Can you work these out from the model? Positions are in its coordinate system, mm. A direction names the side the tool comes from. Give positions to 0.01 mm unless a question says otherwise; leave off trailing zeros. Order: outer loops, then holes, each group sorted by start corner. A loop starts at its lowest first (then second) coordinate and runs counter-clockwise, first axis right, second up.
Item 1: If I drill on line 1 along X through (y, z) = (2.85, -114.5); line 2 along Z through (x, y) = (2.25, -0.5); line 3 along X through (y, z) = (3, -115.5), over which ranges is the centre line in solid material (lowest first)?
Item 2: I'm going to push flat-ended pins straight in: pin 1 Ø1.8 at (x, z) = (6, -114.5) entering from -Y; pin 2 Ø4 at (x, z) = (3, -114) entering from -Y; pin 3 Ø1.6 at (x, y) = (4, 1) entering from -Z; pin 4 Ø0.8 at (x, z) = (5, -109.5) entering from -Y. Where does each tip first touch, or does it pass through?
Item 3: I want a section at D-D, the plane z = -114.5. Write out the boundary of the cut face in (x, y).
Item 4: I want a section at A-A, the plane x = 0. Write out the boundary of the cut face in (y, z), then the cut area to 3 significant figures.
Item 5: If we mould it in two halves opening along X, with no side actions, what happens to faces 1 (the flat face through (3, 4, -113)), 2 (the flat face through (-3, 1.2, -109.5)), 3 (the cylindrical face through (0, 3, -115.6)), 4 (the flat face through (9, 1.2, -109.5))? For each: +X half, -X half, draft (parallel to the pull), parting line (faces both ways), or undercut.
Item 6: I want a section at B-B, the plane y = -0.5. Write out the boundary of the cut face in (x, z).
Item 7: I want a section at C-C, the plane x = 3.5. Write out the boundary of the cut face in (y, z), then the cut area to 3 significant figures.
Item 8: Which directions (+Z, -Z, +X, -X, +Y, -Y) give clear straight access to the entire face, cutting with the end or side of a thin tool? Please do faces 5 (the flat face through (3, 3, -106.5)), 6 (the flat face through (3, 2, -114)), 7 (the cylindrical face through (2.916, 0.432, -106.985)).
```python
from build123d import *

# Parameters (mm, degrees)
SKETCH_1_W                      = 9.5
SKETCH_1_H                      = 13.25
EXTRUDE_1_DEPTH                 = 2
EXTRUDE_2_DEPTH                 = 12
PATTERN_LINEAR_1_COUNT          = 5
PATTERN_LINEAR_1_PITCH          = 22
HOLE_WIZARD_2_2_2_2_1_D         = 2.1
EXTRUDE_3_DEPTH                 = 12
SKETCH_7_W                      = 1.05
SKETCH_7_H                      = 15
EXTRUDE_4_DEPTH                 = 110
HOLE_WIZARD_2_0_2_2_D           = 2
HOLE_WIZARD_2_0_2_2_ON_FACE_2_D = 2
CUT_EXTRUDE_1_DEPTH             = 135.480746763
CUT_EXTRUDE_1_DEPTH_BACK        = 135.480746763
SKETCH_14_W                     = 52.846717088
SKETCH_14_H                     = 8
SKETCH19_W                      = 12
SKETCH19_H                      = 12
EXTRUDE23_DEPTH                 = 2
SKETCH20_R                      = 1.1
EXTRUDE24_DEPTH                 = 2
CUT_EXTRUDE_2_DEPTH             = 22
CUT_EXTRUDE_2_DEPTH_BACK        = 24
SKETCH_15_W                     = 124.248356878
SKETCH_15_H                     = 108.553418936
CUT_EXTRUDE_START               = -90
CUT_EXTRUDE_3_DEPTH             = 90
CUT_EXTRUDE_4_DEPTH             = 18
CUT_EXTRUDE_4_DEPTH_BACK        = 16
SKETCH_18_W                     = 34.927969389
SKETCH_18_H                     = 20.970488767


with BuildPart() as part:
    # 草图1 → 凸台-拉伸1 (new body)
    with BuildSketch(Plane(origin=(0, 0, 0), x_dir=(1, 0, 0), z_dir=(0, 1, 0))):
        Polygon((21.5, 0), (21.5, 110), (9, 110), (0, 101), (0, 0), align=None)
        Polygon((19.121320344, 101), (4.242640687, 101), (8.121320344, 104.878679656), (19.121320344, 104.878679656), align=None, mode=Mode.SUBTRACT)
        with Locations((10.75, 12.625)):
            Rectangle(SKETCH_1_W, SKETCH_1_H, mode=Mode.SUBTRACT)
        with Locations((10.75, 37.875)):
            Rectangle(SKETCH_1_W, SKETCH_1_H, mode=Mode.SUBTRACT)
        with Locations((10.75, 63.125)):
            Rectangle(SKETCH_1_W, SKETCH_1_H, mode=Mode.SUBTRACT)
        with Locations((10.75, 88.375)):
            Rectangle(SKETCH_1_W, SKETCH_1_H, mode=Mode.SUBTRACT)
    extrude(amount=EXTRUDE_1_DEPTH)

    # 草图2 → 凸台-拉伸2 (add)
    with BuildSketch(Plane(origin=(0, 0, -101), x_dir=(-1, 0, 0), z_dir=(0, 0, -1))):
        with BuildLine():
            Line((0, 2), (0, 0))
            Line((0, 0), (3.5, 0))
            ThreePointArc((3.5, 0), (5.08113883, 4.436491673), (1.050510257, 2))
            Line((1.050510257, 2), (0, 2))
        make_face()
    extrude_2 = extrude(amount=-EXTRUDE_2_DEPTH)

    # 阵列(线性)1: 凸台-拉伸2 ×5
    with Locations(*[(0, 0, i * PATTERN_LINEAR_1_PITCH) for i in range(1, PATTERN_LINEAR_1_COUNT)]):
        add(extrude_2)

    # Ø2.2 (2.2) 直径孔1 (through all)
    with Locations(Plane(origin=(0, 0, -101), x_dir=(-1, 0, 0), z_dir=(0, 0, -1))):
        with Locations((3.5, 2.5)):
            Hole(HOLE_WIZARD_2_2_2_2_1_D / 2)

    # 草图5 → 凸台-拉伸3 (add)
    with BuildSketch(Plane(origin=(9, 0, 0), x_dir=(0, 0, -1), z_dir=(1, 0, 0))):
        with BuildLine():
            Line((108.949489743, 0), (110, 0))
            Line((110, 0), (110, 2))
            Line((110, 2), (106.5, 2))
            ThreePointArc((106.5, 2), (104.91886117, -2.436491673), (108.949489743, 0))
        make_face()
    extrude(amount=-EXTRUDE_3_DEPTH)

    # 草图7 → Ø2.2 (2.2) 直径孔2 (revolve, cut)
    with BuildSketch(Plane(origin=(9, -0.5, -106.5), x_dir=(0, 0, -1), z_dir=(0, 1, 0))):
        with Locations((0.525, 7.5)):
            Rectangle(SKETCH_7_W, SKETCH_7_H)
    revolve(axis=Axis((15.35, -0.5, -106.5), (-1, 0, 0)), mode=Mode.SUBTRACT)

    # 草图8 → 凸台-拉伸4 (add)
    with BuildSketch(Plane.XY):
        with BuildLine():
            ThreePointArc((31.5, 0), (34.178784027, 0.532843272), (36.449747468, 2.050252532))
            Line((36.449747468, 2.050252532), (39.577164466, 5.17766953))
            ThreePointArc((39.577164466, 5.17766953), (57.254833996, 12.5), (74.932503526, 5.17766953))
            Line((74.932503526, 5.17766953), (76.346717088, 6.591883092))
            ThreePointArc((76.346717088, 6.591883092), (57.254833996, 14.5), (38.162950904, 6.591883092))
            Line((38.162950904, 6.591883092), (35.035533906, 3.464466094))
            ThreePointArc((35.035533906, 3.464466094), (33.413417162, 2.380602337), (31.5, 2))
            Line((31.5, 2), (21.5, 2))
            Line((21.5, 2), (21.5, 0))
            Line((21.5, 0), (31.5, 0))
        make_face()
    extrude(amount=-EXTRUDE_4_DEPTH)

    # Ø2.0 (2) 直径孔2 (through all)
    with Locations(Plane(origin=(66.489377866, 12.871700761, -5), x_dir=(0.939692620786, -0.342020143326, 0), z_dir=(0.342020143326, 0.939692620786, 0))):
        with Locations((0, 0)):
            Hole(HOLE_WIZARD_2_0_2_2_D / 2)

    # Ø2.0 (2) 直径孔2 on face 2 (through all)
    with Locations(Plane(origin=(66.489377866, 12.871700761, -52), x_dir=(0.939692711209, -0.342019894889, 0), z_dir=(0.342019894889, 0.939692711209, 0))):
        with Locations((0, 0)):
            Hole(HOLE_WIZARD_2_0_2_2_ON_FACE_2_D / 2)

    # 草图14 → 切除-拉伸1 (cut, two sides: drawn at the far end of the back side and taken through both)
    with BuildSketch(Plane(origin=(0, 2, 0), x_dir=(1, 0, 0), z_dir=(0, 1, 0)).offset(-CUT_EXTRUDE_1_DEPTH_BACK)):
        with BuildLine():
            add(Edge.make_bspline(
                [(65.543349365, 5), (65.543349365, 4.867858182), (65.568139282, 4.738193315), (65.663651177, 4.49599396), (65.734288369, 4.385069362), (65.909329104, 4.20058787), (66.014984918, 4.126085586), (66.242291721, 4.026337096), (66.366299142, 4.000069682), (66.611454679, 3.999930602), (66.734292904, 4.025809235), (66.960669981, 4.125923854), (67.063423157, 4.199243917), (67.237262204, 4.385832013), (67.305425299, 4.495895945), (67.398649167, 4.738239585), (67.422691544, 4.869119898), (67.422777552, 5.130169285), (67.398544475, 5.261724961), (67.306168595, 5.502477284), (67.237041074, 5.614131138), (67.065581718, 5.798710334), (66.962099904, 5.873181003), (66.736029766, 5.973681753), (66.61428089, 5.999865952), (66.366377399, 6.000133023), (66.24402893, 5.974291959), (66.014886358, 5.874003493), (65.90992169, 5.799906628), (65.647004042, 5.52319771), (65.543349365, 5.264283637), (65.543349365, 5)],
                knots=[0, 0, 0, 0, 0.0625, 0.0625, 0.125, 0.125, 0.1875, 0.1875, 0.25, 0.25, 0.3125, 0.3125, 0.375, 0.375, 0.4375, 0.4375, 0.5, 0.5, 0.5625, 0.5625, 0.625, 0.625, 0.6875, 0.6875, 0.75, 0.75, 0.8125, 0.8125, 0.875, 0.875, 1, 1, 1, 1], degree=3))
        make_face()
        with Locations((46.923358544, 14)):
            Rectangle(SKETCH_14_W, SKETCH_14_H)
        with Locations((46.923358544, 61)):
            Rectangle(SKETCH_14_W, SKETCH_14_H)
    extrude(amount=CUT_EXTRUDE_1_DEPTH + CUT_EXTRUDE_1_DEPTH_BACK, mode=Mode.SUBTRACT)

    # Sketch19 → Extrude23 (add)
    with BuildSketch(Plane(origin=(0, 2, 0), x_dir=(1, 0, 0), z_dir=(0, 1, 0))):
        with Locations((3, 112.5)):
            Rectangle(SKETCH19_W, SKETCH19_H)
    extrude(amount=EXTRUDE23_DEPTH)

    # Sketch20 → Extrude24 (cut)
    with BuildSketch(Plane(origin=(0, 2, 0), x_dir=(-1, 0, 0), z_dir=(0, -1, 0))):
        with Locations(Location((-6, 114.5, 0), (0, 0, 90))):
            Circle(SKETCH20_R)
        with Locations(Location((0, 114.5, 0), (0, 0, 270))):
            Circle(SKETCH20_R)
    extrude(amount=-EXTRUDE24_DEPTH, mode=Mode.SUBTRACT)

    # 草图15 → 切除-拉伸2 (cut, two sides: drawn at the far end of the back side and taken through both)
    with BuildSketch(Plane(origin=(0, 2, 0), x_dir=(1, 0, 0), z_dir=(0, 1, 0)).offset(-CUT_EXTRUDE_2_DEPTH_BACK)):
        with Locations((56.124178439, 46.723290532)):
            Rectangle(SKETCH_15_W, SKETCH_15_H)
    extrude(amount=CUT_EXTRUDE_2_DEPTH + CUT_EXTRUDE_2_DEPTH_BACK, mode=Mode.SUBTRACT)

    # 草图17 → 切除-拉伸3 (cut)
    with BuildSketch(Plane.ZY.offset(3).offset(CUT_EXTRUDE_START)):
        with BuildLine():
            Line((-106.5, 2), (-106.5, 4))
            Line((-106.5, 4), (-110, 4))
            Line((-110, 4), (-110, 14.5))
            Line((-110, 14.5), (-101, 14.5))
            Line((-101, 14.5), (-101, 0))
            Line((-101, 0), (-104.050510257, 0))
            ThreePointArc((-104.050510257, 0), (-104.91886117, 1.436491673), (-106.5, 2))
        make_face()
    extrude(amount=CUT_EXTRUDE_3_DEPTH, mode=Mode.SUBTRACT)

    # 草图18 → 切除-拉伸4 (cut, two sides: drawn at the far end of the back side and taken through both)
    with BuildSketch(Plane(origin=(0, 4, 0), x_dir=(1, 0, 0), z_dir=(0, 1, 0)).offset(-CUT_EXTRUDE_4_DEPTH_BACK)):
        with Locations((26.463984695, 108.014755617)):
            Rectangle(SKETCH_18_W, SKETCH_18_H)
    extrude(amount=CUT_EXTRUDE_4_DEPTH + CUT_EXTRUDE_4_DEPTH_BACK, mode=Mode.SUBTRACT)


solid = part.part
```
Results list:
1. line 1: x = -3 to -1.1, 1.1 to 4.9, 7.1 to 9
1. line 2: z = -109 to -107.55, -105.45 to -104
1. line 3: x = -3 to -0.46, 0.46 to 5.54, 6.46 to 9
2. pin 1: passes through
2. pin 2: stops at y = 2
2. pin 3: stops at z = -110
2. pin 4: stops at y = 0
3. outline: (-3, 2) - (-1.1, 2) - (-1.1, 4) - (-3, 4) - close; (1.1, 2) - (4.9, 2) - (4.9, 4) - (1.1, 4) - close; (7.1, 2) - (9, 2) - (9, 4) - (7.1, 4) - close
4. outline: (0, -110) - (2, -110) - (2, -113.4) - (4, -113.4) - (4, -106.5) - (2, -106.5) arc R2.5 ccw (long way) to (0, -108.95) - close; (2, -118.5) - (4, -118.5) - (4, -115.6) - (2, -115.6) - close; hole circle Ø2.1 at (-0.5, -106.5)
4. area: 39.1 mm2
5. face 1: draft
5. face 2: -X half
5. face 3: undercut
5. face 4: +X half
6. outline: (-3, -109) - (9, -109) - (9, -107.55) - (-3, -107.55) - close; (-3, -105.45) - (9, -105.45) - (9, -104) - (-3, -104) - close
7. outline: (0, -110) - (2, -110) - (2, -118.5) - (4, -118.5) - (4, -106.5) - (2, -106.5) arc R2.5 ccw (long way) to (0, -108.95) - close; hole circle Ø2.1 at (-0.5, -106.5)
7. area: 43.5 mm2
8. face 5: +Z, +X, -X, +Y
8. face 6: -Z, +X, -X, -Y
8. face 7: +X, -X
